Can you work these out from the model? Positions are in its coordinate system, mm. Face numbers are marked on the shaded views. A direction names the side the tool comes from. Coordinates: 2 decimals unless noted, no trailing zeros. Loops run counter-clockwise (first coordinate to the right, second up) from the corner with the lowest first, then second, coordinate; pieces in that order, holes last. Notation, with made-up numbers: (-22, 73) -> (1, 73) arc R38 ccw to (1, 111) -> close; hole circle Ø2 at (10.5, -31). An arc over 180 degrees is marked (long way). Put each result on its own line as item: value. Start each with the question number.
Item 1: If we section it at D-D on z = 4.25: Please give me the cut outline in (x, y).
Item 2: We'd pull the mould along Y, two halves only. Please class the marked faces 1, 2 and 3: pulls with the +Y half, pulls with the -Y half, needs draft (parallel to the pull), parting line crosses it, or undercut.
Item 3: Will these pins go through, and if not, where does the flat tip stop? P1, Ø9, axis at x = 0, y = 24, coming from the +Z side; P2, Ø4.5, axis at x = 14.11, y = -19.42, coming from the -Z side; P3, Ø1.5, axis at x = 7, z = 5.5, coming from the -Y side; P4, Ø5, axis at x = -20.5, z = 6.5, coming from the -Y side.
Item 4: If we section it at C-C on y = 0: Please give me the cut outline in (x, z), plus the area to 3 significant figures.
Item 5: For the marked faces 4 and 5, which set-ups out of +Z, -Z, +X, -X, +Y, -Y let a thin tool reach every point of the face, with its end or its side?
Item 6: If we section it at B-B on z = 7.75: State how many separate pieces and enclosed holes the cut face has, plus the area to 3 significant figures.
Item 7: If we section it at A-A on x = 0: Please give me the cut outline in (y, z).
Item 8: Please list where these lines run through material, in increasing order: L1, parallel to Y at x = 0, z = 6.85; L2, parallel to X at y = -21, z = 10; L3, parallel to X at y = 6, z = 3.25. Write a range as from..to.
```python
from build123d import *

# Parameters (mm, degrees)
F0_R     = 11.5
F1_DEPTH = 15
F0_R_2   = 14.5
F2_DEPTH = 5
F0_R_3   = 32
F3_DEPTH = 11
F4_D     = 5.5
F5_D     = 8.8
F6_SIZE  = 1
F7_SIZE  = 1
F8_SIZE  = 1


with BuildPart() as f1:
    # F0 (on Top) → F1 (new body)
    with BuildSketch(Plane.XY):
        Circle(F0_R)
    extrude(amount=F1_DEPTH)

    # F0 (on Top) → F2 (join)
    with BuildSketch(Plane.XY):
        Circle(F0_R_2)
        Circle(F0_R, mode=Mode.SUBTRACT)
    extrude(amount=F2_DEPTH)

    # F0 (on Top) → F3 (join)
    with BuildSketch(Plane.XY):
        Circle(F0_R_3)
        Circle(F0_R_2, mode=Mode.SUBTRACT)
    extrude(amount=F3_DEPTH)

    # F4 (through all)
    with Locations(Plane(origin=(0, 0, 0), x_dir=(1, 0, 0), z_dir=(0, 0, -1))):
        with Locations((-22.8253563911, -7.416407865), (0, -24), (22.8253563911, -7.416407865), (14.106846055, 19.416407865), (-14.106846055, 19.416407865)):
            Hole(F4_D / 2)

    # F5 (through all)
    with Locations(Plane(origin=(0, 0, 0), x_dir=(1, 0, 0), z_dir=(0, 0, -1))):
        with Locations((0, 0)):
            Hole(F5_D / 2)

    # F6
    f6_edges = [f1.edges().sort_by_distance(p)[0] for p in [
        (-11.5, 0, 15),
    ]]
    chamfer(f6_edges, length=F6_SIZE)

    # F7
    f7_edges = [f1.edges().sort_by_distance(p)[0] for p in [
        (-14.5, 0, 11),
    ]]
    chamfer(f7_edges, length=F7_SIZE)

    # F8
    f8_edges = [f1.edges().sort_by_distance(p)[0] for p in [
        (-32, 0, 11),
    ]]
    chamfer(f8_edges, length=F8_SIZE)


solid = f1.part
```
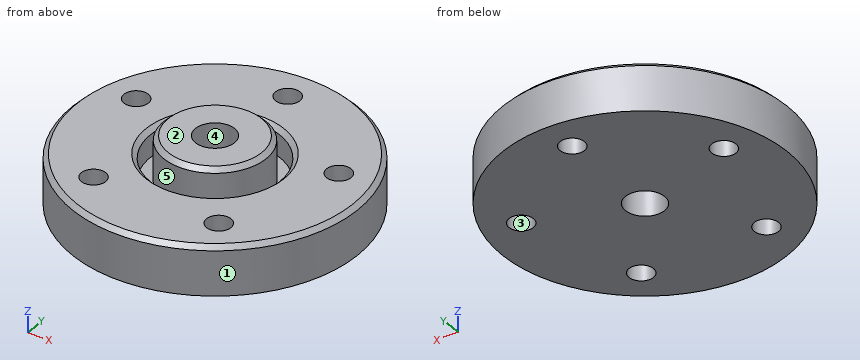
Solutions:
1. outline: circle Ø64 at (0, 0); hole circle Ø5.5 at (-22.83, 7.42); hole circle Ø5.5 at (-14.11, -19.42); hole circle Ø8.8 at (0, 0); hole circle Ø5.5 at (0, 24); hole circle Ø5.5 at (14.11, -19.42); hole circle Ø5.5 at (22.83, 7.42)
2. face 1: parting line crosses it
2. face 2: needs draft
2. face 3: undercut
3. P1: z = 11
3. P2: through
3. P3: y = -31.38
3. P4: y = -26.46
4. outline: (-32, 0) -> (-4.4, 0) -> (-4.4, 15) -> (-10.5, 15) -> (-11.5, 14) -> (-11.5, 5) -> (-14.5, 5) -> (-14.5, 10) -> (-15.5, 11) -> (-31, 11) -> (-32, 10) -> close; (4.4, 0) -> (32, 0) -> (32, 10) -> (31, 11) -> (15.5, 11) -> (14.5, 10) -> (14.5, 5) -> (11.5, 5) -> (11.5, 14) -> (10.5, 15) -> (4.4, 15) -> close
4. area: 625 mm^2
5. face 4: +Z, -Z
5. face 5: +Z
6. separate pieces: 2
6. enclosed holes: 7
6. area: 2,790 mm^2
7. outline: (-32, 0) -> (-4.4, 0) -> (-4.4, 15) -> (-10.5, 15) -> (-11.5, 14) -> (-11.5, 5) -> (-14.5, 5) -> (-14.5, 10) -> (-15.5, 11) -> (-31, 11) -> (-32, 10) -> close; (4.4, 0) -> (21.25, 0) -> (21.25, 11) -> (15.5, 11) -> (14.5, 10) -> (14.5, 5) -> (11.5, 5) -> (11.5, 14) -> (10.5, 15) -> (4.4, 15) -> close; (26.75, 0) -> (32, 0) -> (32, 10) -> (31, 11) -> (26.75, 11) -> close
8. L1: -32..-14.5, -11.5..-4.4, 4.4..11.5, 14.5..21.25, 26.75..32
8. L2: -24.15..-16.36, -11.86..11.86, 16.36..24.15
8. L3: -31.43..-25.18, -20.47..20.47, 25.18..31.43
